from build123d import *

# Parameters (mm, degrees)
F1_DEPTH = 4
F2_D     = 3


with BuildPart() as f1:
    # F0 (on Top) → F1 (new body)
    with BuildSketch(Plane.XY):
        Polygon((0, 0), (-114.5, 225), (-229, 0), (-229, -25), (0, -25), align=None)
    extrude(amount=F1_DEPTH)

    # F2 (through all)
    with Locations(Plane(origin=(0, 0, 0), x_dir=(1, 0, 0), z_dir=(0, 0, -1))):
        with Locations((-114.5, -214), (-219, -5), (-146.5, 0), (-146.5, 20), (-86.5, 20), (-86.5, 0), (-10, -5)):
            Hole(F2_D / 2)


solid = f1.part
Input: part model. Units: mm. Frame: model coordinates. Give positions to 0.01 mm unless a question says otherwise; leave off trailing zeros. Write each loop counter-clockwise with the first axis right and the second up, starting at its lowest first coordinate (ties: lowest second). Pieces come first, ordered by that corner, then holes.
Q1. Section A-A, the plane z = 1.8. Output: boundary loops of the cut face in (x, y).
Q2. Section B-B, the plane x = -75. Output: boundary loops of the cut face in (y, z).
Q3. Section C-C, the plane y = 208. Output: boundary loops of the cut face in (x, z), plus the area to 3 significant figures.
Q4. Material intervals for probe 1 along X at (y, z) = (-20, 2.3); probe 2 along Y at (x, z) = (-114.5, 2.15); probe 3 along Y at (x, z) = (-146.5, 2.05), sorted ascending.
Q5. First-contact query: P1, Ø2.5, axis at x = -86.5, y = 0, coming from the -Z side; P2, Ø5, axis at x = -86.5, y = -20, coming from the -Z side; P3, Ø2, axis at x = -185.5, z = 3, coming from the +Y side; P4, Ø2, axis at y = 189, z = 3, coming from the -X side. Flat tips, straight axial feed; report the tip coordinate or a pass-through.
Filled in:
1. outline: (-229, -25) - (0, -25) - (0, 0) - (-114.5, 225) - (-229, 0) - close; hole circle Ø3 at (-219, 5); hole circle Ø3 at (-146.5, -20); hole circle Ø3 at (-146.5, 0); hole circle Ø3 at (-114.5, 214); hole circle Ø3 at (-86.5, -20); hole circle Ø3 at (-86.5, 0); hole circle Ø3 at (-10, 5)
2. outline: (-25, 0) - (147.38, 0) - (147.38, 4) - (-25, 4) - close
3. outline: (-123.15, 0) - (-105.85, 0) - (-105.85, 4) - (-123.15, 4) - close
3. area: 69.2 mm2
4. probe 1: x = -229 to -148, -145 to -88, -85 to 0
4. probe 2: y = -25 to 212.5, 215.5 to 225
4. probe 3: y = -25 to -21.5, -18.5 to -1.5, 1.5 to 162.12
5. P1: passes through
5. P2: stops at z = 0
5. P3: stops at y = 87.45
5. P4: stops at x = -133.33
